```python
from build123d import *

# Parameters (mm, degrees)
F0_W      = 55.5363558233
F0_H      = 30
F1_DEPTH  = 17.5
F1_FACE_W = 55.5363558233
F1_FACE_H = 35
F2_DEPTH  = 30
F2_TAPER  = 5
F3_R      = 12.5
F4_DEPTH  = 50
F4_TAPER  = -6
F6_DEPTH  = 35
F8_DEPTH  = 35


with BuildPart() as f1:
    # F0 (on Front) → F1 (new body, symmetric)
    with BuildSketch(Plane.XZ):
        with Locations((27.7681779116, 15)):
            Rectangle(F0_W, F0_H)
    extrude(amount=F1_DEPTH, both=True)

    # F1_face (on face) → F2 (join)
    with BuildSketch(Plane(origin=(27.7681779116, 0, 0), x_dir=(1, 0, 0), z_dir=(0, 0, -1))):
        Rectangle(F1_FACE_W, F1_FACE_H)
    extrude(amount=F2_DEPTH, taper=F2_TAPER)

    # F3 (on face) → F4 (join)
    with BuildSketch(Plane(origin=(0, 0, 0), x_dir=(0, -1, 0), z_dir=(-1, 0, 0))):
        with Locations((0, 15)):
            Circle(F3_R)
    extrude(amount=F4_DEPTH, taper=F4_TAPER)

    # F5 (on face) → F6 (join)
    with BuildSketch(Plane.XZ.offset(17.5)):
        with BuildLine():
            ThreePointArc((120, 0), (87.9580104682, 22.8252746923), (49.2771938443, 30))
            Line((49.2771938443, 30), (49.2771938443, 15))
            ThreePointArc((49.2771938443, 15), (86.0226572611, 14.0256420707), (120, 0))
        make_face()
    extrude(amount=-F6_DEPTH)

    # F7 (on face) → F8 (cut)
    with BuildSketch(Plane.XY.offset(30)):
        Polygon((147.9074739632, 6.4577797765), (56.5133458154, 2.4674259652), (56.5133458154, -2.4674259652), (147.8689167317, -6.4560963314), align=None)
    extrude(amount=-F8_DEPTH, mode=Mode.SUBTRACT)


solid = f1.part
```
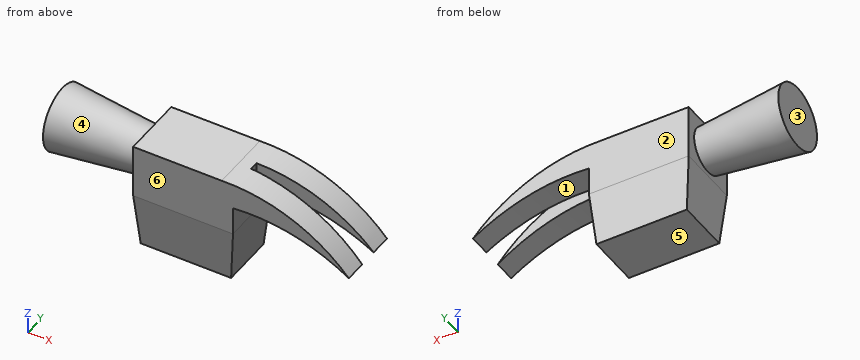
Check sheet for the modelled part. Datum: model origin and axes. Units: mm. Face numbers are marked on the shaded views. A direction names the side the tool comes from. Round coordinates to 2 decimals unless told otherwise and drop trailing zeros. Loops run counter-clockwise (first coordinate to the right, second up) from the corner with the lowest first, then second, coordinate; pieces in that order, holes last. Notation, with made-up numbers: (-3.5, -22.75) - (5.5, -22.75) arc R20 cw to (5.5, -11.75) - close; hole circle Ø8 at (51.5, 72). An arc over 180 degrees is marked (long way). Write item = value, one per line. Start each with the question number.
Q1. Section check A-A (x = -17). Record the boundary of the cut face in (y, z).
Q2. Release check for a two-part mould opening along X. For the marked faces 1, 2, 3 and 4 record: pulls with the +X half, pulls with the -X half, needs draft (parallel to the pull), parting line crosses it, or undercut.
Q3. Access from +Z, -Z, +X, -X, +Y, -Y to the whole of each face (thin tool, end or side, straight path). Record for the marked faces 5 and 6.
Q4. Thickness scan on L1, parallel to Z at x = 57, y = 16; L2, parallel to Y at x = 73, z = 16.5; L3, parallel to Y at x = 6, z = 12. Record the ranges inside material, lowest first.
Q5. Depth check by flat-ended pin: P1, Ø8, axis at x = 58.5, z = -18.5, coming from the -Y side; P2, Ø10, axis at y = 14, z = -10, coming from the +X side; P3, Ø1, axis at x = 10, z = 13.5, coming from the -Y side; P4, Ø15, axis at x = 57.5, z = 10.5, coming from the +Y side. Enter the tip coordinate at first touch or a pass-through.
Derived:
q1.outline = circle Ø28.57 at (0, 15)
q2.face_1 = undercut
q2.face_2 = needs draft
q2.face_3 = pulls with the -X half
q2.face_4 = undercut
q3.face_5 = -Z, +X, -X, +Y, -Y
q3.face_6 = +Z, -Z, +X, -Y
q4.L1 = 15.91 to 29.94
q4.L2 = -17.5 to -3.19, 3.19 to 17.5
q4.L3 = -17.5 to 17.5
q5.P1 = through
q5.P2 = 55.1
q5.P3 = -17.5
q5.P4 = 17.5
